from build123d import *

# Parameters (mm, degrees)
SKETCH_1_R      = 12.2
EXTRUDE_1_DEPTH = 51.8
SKETCH_5_R      = 3.5
EXTRUDE_3_DEPTH = 2.5
SKETCH_6_R      = 2
EXTRUDE_4_DEPTH = 8


with BuildPart() as part:
    # 草图1 → 凸台-拉伸1 (new body)
    with BuildSketch(Plane.XY):
        with Locations(Location((0, 0, 0), (0, 0, 180))):
            Circle(SKETCH_1_R)
    extrude(amount=EXTRUDE_1_DEPTH)

    # 草图5 → 凸台-拉伸3 (add)
    with BuildSketch(Plane.XY.offset(51.8)):
        Circle(SKETCH_5_R)
    extrude(amount=EXTRUDE_3_DEPTH)

    # 草图6 → 凸台-拉伸4 (add)
    with BuildSketch(Plane.XY.offset(54.3)):
        Circle(SKETCH_6_R)
    extrude(amount=EXTRUDE_4_DEPTH)


solid = part.part
Could you check a few things on this model? Use its own coordinates, in mm. A direction names the side the tool comes from. Give positions to 0.01 mm unless a question says otherwise; leave off trailing zeros. Order: outer loops, then holes, each group sorted by start corner. A loop starts at its lowest first (then second) coordinate and runs counter-clockwise, first axis right, second up.
1. Suppose I cut it at A-A (x = 0). List the corners of the cut face in (y, z) for me, plus the area to 3 significant figures.
2. I need wall thicknesses on L1, parallel to Z at x = 3, y = -3.5; L2, parallel to Y at x = -0.5, z = 49.5; L3, parallel to X at y = 11, z = 38.5. Which ranges of each line are inside material? Lowest first, please.
3. Will these pins go through, and if not, where does the flat tip stop? P1, Ø4, axis at x = -8, z = 9, coming from the +Y side; P2, Ø1, axis at y = 6, z = 7, coming from the +X side; P3, Ø1.5, axis at x = 0.5, y = 9, coming from the +Z side.
4. For faces 1 (the flat face through (0, 0, 62.3)), 2 (the flat face through (2, -2, 54.3)), which set-ups out of +Z, -Z, +X, -X, +Y, -Y let a thin tool reach every point of the face, with its end or its side?
5. Suppose I cut it at D-D (y = -7.5). List the corners of the cut face in (x, z) for me.
6. Suppose I cut it at C-C (z = 42.5). List the corners of the cut face in (x, y) for me.
Solved:
1. outline: (-12.2, 0) - (12.2, 0) - (12.2, 51.8) - (3.5, 51.8) - (3.5, 54.3) - (2, 54.3) - (2, 62.3) - (-2, 62.3) - (-2, 54.3) - (-3.5, 54.3) - (-3.5, 51.8) - (-12.2, 51.8) - close
1. area: 1,310 mm2
2. L1: z = 0 to 51.8
2. L2: y = -12.19 to 12.19
2. L3: x = -5.28 to 5.28
3. P1: stops at y = 10.62
3. P2: stops at x = 10.89
3. P3: stops at z = 51.8
4. face 1: +Z, +X, -X, +Y, -Y
4. face 2: +Z
5. outline: (-9.62, 0) - (9.62, 0) - (9.62, 51.8) - (-9.62, 51.8) - close
6. outline: circle Ø24.4 at (0, 0)
